Part model, mm, in its own coordinate system. Give positions to 0.01 mm unless a question says otherwise; leave off trailing zeros. Order: outer loops, then holes, each group sorted by start corner. A loop starts at its lowest first (then second) coordinate and runs counter-clockwise, first axis right, second up. Notation, with made-up numbers: (-13, -38.5) - (29, -38.5) arc R17 cw to (29, -17.5) - close; hole circle Ø9 at (-30.5, 55.25). An arc over 180 degrees is marked (long way). Use one line per item in the form item = value. Start each with the question number.
1. Drill centre lines: line 1 (X direction, y = 7.5, z = 0.25) (3 decimals); line 2 (X direction, y = 6.25, z = 1.5) (3 decimals); line 3 (X direction, y = 13.25, z = 0.8) (3 decimals). Where is each one in solid material? Low to high.
2. Pin check, flat tip, straight feed: P1, Ø6.5, axis at x = -40.16, y = 19.41, coming from the -Z side. Stop position of the tip, or through.
3. Band-saw the part on A-A, the plane y = 14.5. List the corners of the cut face in (x, z) (3 decimals).
4. Band-saw the part on B-B, the plane z = 1.4. List the corners of the cut face in (x, y) (1 decimal), plus the area to 3 significant figures.
5. Pull direction X, two halves, no side cores. Call faces 1 (the face through (48.835, 14, 1)), 2 (the face through (47.743, 8.512, 1.014)), 3 (the face through (3, 3.912, 1)): +X half, -X half, draft (parallel to the pull), parting line (faces both ways), or undercut.
Autodesk Inventor part; units mm, degrees
ref_plane "YZ Plane" through (0, 0, 0) normal (1, 0, 0) x (0, 1, 0)
ref_plane "XZ Plane" through (0, 0, 0) normal (0, 1, 0) x (-1, 0, 0)
ref_plane "XY Plane" through (0, 0, 0) normal (0, 0, 1) x (1, 0, 0)
sketch "Эскиз1" plane through (0, 0, 0) normal (0, 0, 1) x (1, 0, 0)
  line L0 (-43.165, 23.4115) -> (48.835, 23.4115)
  line L1 (48.835, 23.4115) -> (48.835, 3.9115)
  line L2 (48.835, 3.9115) -> (-43.165, 3.9115)
  line L3 (-43.165, 3.9115) -> (-43.165, 23.4115)
  point P0 (0, 0)
  dimension "d0" = 92
  dimension "d1" = 19.5
extrude "Выдавливание1" add sketch "Эскиз1" along normal blind 2
sketch "Эскиз2" plane through (0, 0, 2) normal (0, 0, 1) x (1, 0, 0)
  circle A0 centre (-40.165, 7.4115) radius 2
  line L0 (-43.165, 23.4115) -> (-43.165, 3.9115)
  line L1 (-43.165, 3.9115) -> (48.835, 3.9115)
  circle A1 centre (-40.165, 19.4115) radius 2
  line L2 (48.835, 23.4115) -> (-43.165, 23.4115)
  circle A2 centre (45.835, 19.9115) radius 2
  line L3 (48.835, 3.9115) -> (48.835, 23.4115)
  circle A3 centre (45.835, 7.9115) radius 2
  circle A4 centre (2.835, 13.6615) radius 2
  point P0 (0, 0)
  dimension "d4" = 1
  dimension "d5" = 4
  dimension "d6" = 1.5
  dimension "d7" = 4
  dimension "d8" = 1
  dimension "d9" = 2
  dimension "d10" = 4
  dimension "d11" = 1
  dimension "d12" = 1.5
  dimension "d13" = 4
  dimension "d14" = 1
  dimension "d15" = 2
  dimension "d16" = 4
  dimension "d17" = 44
  dimension "d19" = 7.75
extrude "Выдавливание2" cut sketch "Эскиз2" against normal through all contours A0 | A1 | A2 | A3 | A4
properties part number "Пластинка шасси"
From the geometry:
q1.line_1 = -43.165 to -42.163, -38.167 to 43.878, 47.792 to 48.835
q1.line_2 = -43.165 to -41.793, -38.537 to 44.722, 46.948 to 48.835
q1.line_3 = -43.165 to 0.878, 4.792 to 48.835
q2.P1 = 0
q3.outline = (-43.165, 0) - (1.019, 0) - (1.019, 2) - (-43.165, 2) - close; (4.651, 0) - (48.835, 0) - (48.835, 2) - (4.651, 2) - close
q4.outline = (-43.2, 3.9) - (48.8, 3.9) - (48.8, 23.4) - (-43.2, 23.4) - close; hole circle Ø4 at (-40.2, 7.4); hole circle Ø4 at (-40.2, 19.4); hole circle Ø4 at (2.8, 13.7); hole circle Ø4 at (45.8, 7.9); hole circle Ø4 at (45.8, 19.9)
q4.area = 1,730 mm²
q5.face_1 = +X half
q5.face_2 = undercut
q5.face_3 = draft
